Build history of the part. All positions in model axes, mm. Coordinates: 2 decimals unless noted, no trailing zeros. Order: outer loops, then holes, each group sorted by start corner. A loop starts at its lowest first (then second) coordinate and runs counter-clockwise, first axis right, second up. Notation, with made-up numbers: (40, -24) - (74, -24) arc R34 ccw to (74, 13) - close; hole circle Ø5 at (78.5, -6.75). An arc over 180 degrees is marked (long way). Return JSON: item names as keys, results as strings.
from build123d import *

# Parameters (mm, degrees)
F0_R     = 3.1
F1_DEPTH = 14
F2_R     = 4
F3_DEPTH = 25
F5_DEPTH = 25
F6_R     = 12


with BuildPart() as f1:
    # F0 (on Right) → F1 (new body)
    with BuildSketch(Plane.YZ):
        Polygon((36.3872624823, -13.7823516789), (36.3872624823, -6.2581492842), (18.3872624823, -7.7053745112), (-25.0031341377, 17.139614544), (-29.9721319488, 8.46153522), (12.2630268532, -15.7219740336), align=None)
        with Locations((-22.3021764927, 9.8314245335)):
            Circle(F0_R, mode=Mode.SUBTRACT)
        with Locations((-22.3021764927, 9.8314245335)):
            Circle(F0_R)
    extrude(amount=F1_DEPTH)

    # F2 (on face) → F3 (cut)
    with BuildSketch(Plane(origin=(0, 0.733642711, -9.1247502824), x_dir=(1, 0, 0), z_dir=(0, -0.0801427819, 0.996783394))):
        with Locations((7, 26.7105877545)):
            Circle(F2_R)
    extrude(amount=-F3_DEPTH, mode=Mode.SUBTRACT)

    # F4 (on face) → F5 (cut)
    with BuildSketch(Plane(origin=(0, 1.2173257447, 2.1259919559), x_dir=(1, 0, 0), z_dir=(0, 0.4968997811, 0.8678079324))):
        with BuildLine():
            ThreePointArc((3.5, -37.5475101173), (7, -41.0475101173), (10.5, -37.5475101173))
            Line((10.5, -37.5475101173), (10.5, 11.3638080657))
            ThreePointArc((10.5, 11.3638080657), (7, 14.8638080657), (3.5, 11.3638080657))
            Line((3.5, 11.3638080657), (3.5, -37.5475101173))
        make_face()
    extrude(amount=-F5_DEPTH, mode=Mode.SUBTRACT)

    # F6
    f6_edges = [f1.edges().sort_by_distance(p)[0] for p in [
        (7, 18.387262, -7.705375),
        (7, 12.263027, -15.721974),
    ]]
    fillet(f6_edges, radius=F6_R)


solid = f1.part
1. Cut at B-B on x = 9.5. Give the cut face in (y, z).
Check values:
{"outline": "(8.24, -13.42) - (9.04, -13.88) arc R12 ccw to (15.96, -15.42) - (24.85, -14.71) - (24.25, -7.23) - (22.09, -7.41) arc R12 cw to (15.16, -5.86) - (13.2, -4.74) - close; (30.47, -6.73) - (31.07, -14.21) - (36.39, -13.78) - (36.39, -6.26) - close"}
2. Probe L1, parallel to X at y = -4.5, z = -4; L2, parallel to X at y = 10, z = -8; L3, parallel to Y at x = 10.75, z = -3.5. List the from-to ranges inside material, lowest first.
Check values:
{"L1": "0 to 3.5, 10.5 to 14", "L2": "0 to 3.75, 10.25 to 14", "L3": "-9.08 to 11.04"}
3. Drop flat-ended pins along their axis: pin 1 (6 mm diameter, centred on x = 3.5, z = -2.5, fed in from -Y); pin 2 (8 mm diameter, centred on x = 7.5, y = 21, fed in from -Z). Give the stop position or say it passes through.
Check values:
{"pin 1": "y = -16.07", "pin 2": "z = -15.34"}
4. Cut at D-D on x = 5. Give the cut face in (y, z), plus the area to 3 significant figures.
Check values:
{"outline": "(8.6, -13.63) - (9.04, -13.88) arc R12 ccw to (15.96, -15.42) - (24.51, -14.74) - (23.91, -7.26) - (22.09, -7.41) arc R12 cw to (15.16, -5.86) - (13.57, -4.95) - close; (30.81, -6.71) - (31.41, -14.18) - (36.39, -13.78) - (36.39, -6.26) - close", "area": "155 mm²"}
5. Cut at C-C on z = 7. Give the cut face in (x, y), plus the area to 3 significant figures.
Check values:
{"outline": "(0, -27.42) - (3.5, -27.42) - (3.5, -7.29) - (0, -7.29) - close; (10.5, -27.42) - (14, -27.42) - (14, -7.29) - (10.5, -7.29) - close", "area": "141 mm²"}
6. Mould opens along Y. For faces 1 (the cylindrical face through (3.004, 27.83, -10.656)), 2 (the flat face through (6.9, 32.52, -6.57)), 3 (the flat face through (1.726, -27.453, 12.861)), 4 (the flat face through (6.902, 23.763, -14.797)) say: pulls with the +Y half, pulls with the -Y half, needs draft (parallel to the pull), parting line crosses it, or undercut.
Check values:
{"face 1": "undercut", "face 2": "undercut", "face 3": "pulls with the -Y half", "face 4": "pulls with the +Y half"}
7. Cut at A-A on y = -23.5. Give the cut face in (x, z), plus the area to 3 significant figures.
Check values:
{"outline": "(0, 4.76) - (3.5, 4.76) - (3.5, 16.28) - (0, 16.28) - close; (10.5, 4.76) - (14, 4.76) - (14, 16.28) - (10.5, 16.28) - close", "area": "80.7 mm²"}
